Here's how the part is built. I have some questions about the finished solid (model axes, mm). Face numbers are marked on the shaded views. A direction names the side the tool comes from. Round coordinates to 2 decimals unless told otherwise and drop trailing zeros. Write each loop counter-clockwise with the first axis right and the second up, starting at its lowest first coordinate (ties: lowest second). Pieces come first, ordered by that corner, then holes. Notation, with made-up numbers: (-3.75, 41.25) -> (20.25, 41.25) arc R6 cw to (20.25, 47.25) -> close; hole circle Ø1 at (-4, 13.25). An arc over 180 degrees is marked (long way). Answer as CSV lines item,"result".
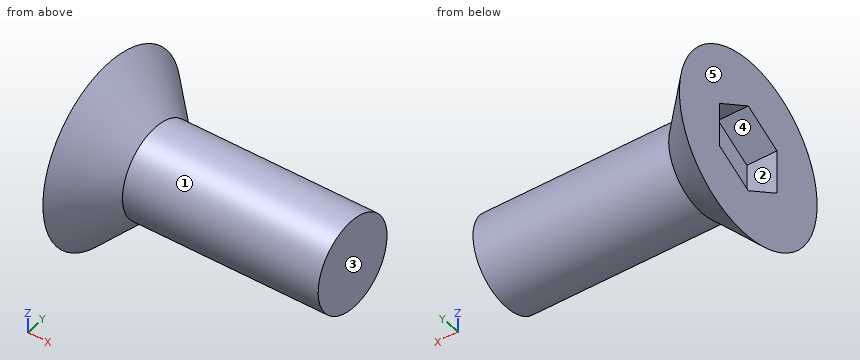
Autodesk Inventor part; units mm, degrees
ref_plane "YZ Plane" through (0, 0, 0) normal (1, 0, 0) x (0, 1, 0)
ref_plane "XZ Plane" through (0, 0, 0) normal (0, 1, 0) x (-1, 0, 0)
ref_plane "XY Plane" through (0, 0, 0) normal (0, 0, 1) x (1, 0, 0)
sketch "Esquisse1" plane through (0, 0, 0) normal (0, 1, 0) x (-1, 0, 0)
  line L0 (0, 0) -> (8, 0)
  line L1 (8, 0) -> (8, -3)
  line L2 (8, -3) -> (6.5, -1.5)
  line L3 (6.5, -1.5) -> (0, -1.5)
  line L4 (0, -1.5) -> (0, 0)
  line L5 (8, 0) -> (8, 3)
  line L6 (8, 3) -> (6.5, 1.5)
  line L7 (6.5, 1.5) -> (0, 1.5)
  line L8 (0, 1.5) -> (0, 0)
  dimension "d0" = 90
  dimension "d1" = 3
  dimension "d2" = 6
  dimension "d3" = 8
revolve "Révolution1" add sketch "Esquisse1" angle 360 about axis through (0, 0, 0) along (-1, 0, 0) contours L0 L1 L2 L3 L4
sketch "Esquisse2" plane through (-8, 0, 0) normal (-1, 0, 0) x (0, 0, 1)
  line L0 (0.7217, 1.25) -> (1.4434, 0)
  line L1 (1.4434, 0) -> (0.7217, -1.25)
  line L2 (0.7217, -1.25) -> (-0.7217, -1.25)
  line L3 (-0.7217, -1.25) -> (-1.4434, 0)
  line L4 (-1.4434, 0) -> (-0.7217, 1.25)
  line L5 (-0.7217, 1.25) -> (0.7217, 1.25)
  point P0 (0, 0)
  point P1 (0, 0)
  dimension "d5" = 2.5
extrude "Extrusion1" cut sketch "Esquisse2" against normal blind 1
properties part number "fraisee"
Item 1: I need wall thicknesses on L1, parallel to X at y = -0.7, z = -0.9; L2, parallel to Y at x = -6, z = -0.4; L3, parallel to X at y = 2.2, z = 1.4. Which ranges of each line are inside material? Lowest first, please.
Results found:
L1,"x = -7 to 0"
L2,"y = -1.45 to 1.45"
L3,"x = -8 to -7.61"
Item 2: For the marked faces 4 and 5, which set-ups out of +Z, -Z, +X, -X, +Y, -Y let a thin tool reach every point of the face, with its end or its side?
Results found:
face 4,"-X"
face 5,"+Z, -Z, -X, +Y, -Y"
Item 3: Suppose I cut it at C-C, the plane x = -1. List the corners of the cut face in (y, z) for me.
Results found:
outline,"circle Ø3 at (0, 0)"
Item 4: Suppose I cut it at A-A, the plane z = 0. List the corners of the cut face in (x, y) for me.
Results found:
outline,"(-8, -3) -> (-6.5, -1.5) -> (0, -1.5) -> (0, 1.5) -> (-6.5, 1.5) -> (-8, 3) -> (-8, 1.25) -> (-7, 1.25) -> (-7, -1.25) -> (-8, -1.25) -> close"
Item 5: Suppose I cut it at B-B, the plane x = -6.75. List the corners of the cut face in (y, z) for me, then the cut area to 3 significant figures.
Results found:
outline,"circle Ø3.5 at (0, 0)"
area,"9.62 mm²"
Item 6: Will these pins go through, and if not, where does the flat tip stop? pin 1 (2 mm diameter, centred on x = -7, z = -2, fed in from -Y); pin 2 (1.1 mm diameter, centred on x = -7.5, z = 0.5, fed in from +Y); pin 3 (1.5 mm diameter, centred on x = -1, y = -1, fed in from +Z).
Results found:
pin 1,"stops at y = -2.44"
pin 2,"stops at y = 2.99"
pin 3,"stops at z = 1.48"
Item 7: If we mould it in two halves opening along Z, with no side actions, what happens to the marked faces 1, 2 and 3? For each: pulls with the +Z half, pulls with the -Z half, needs draft (parallel to the pull), parting line crosses it, or undercut.
Results found:
face 1,"parting line crosses it"
face 2,"undercut"
face 3,"needs draft"
